Autodesk Inventor part; units mm, degrees
ref_plane "YZ Plane" through (0, 0, 0) normal (1, 0, 0) x (0, 1, 0)
ref_plane "XZ Plane" through (0, 0, 0) normal (0, 1, 0) x (-1, 0, 0)
ref_plane "XY Plane" through (0, 0, 0) normal (0, 0, 1) x (1, 0, 0)
sketch "Sketch1" plane through (0, 0, 0) normal (0, 0, 1) x (1, 0, 0)
  line L0 (0, 0) -> (25.4, 0)
  line L1 (25.4, 0) -> (25.4, 50.8)
  line L2 (25.4, 50.8) -> (0, 50.8)
  line L3 (0, 50.8) -> (0, 0)
  line L4 (1.5875, 49.2125) -> (23.8125, 49.2125)
  line L5 (23.8125, 49.2125) -> (23.8125, 1.5875)
  line L6 (23.8125, 1.5875) -> (1.5875, 1.5875)
  line L7 (1.5875, 1.5875) -> (1.5875, 49.2125)
  dimension "d0" = 25.4
  dimension "d1" = 50.8
  dimension "d2" = 1.5875
extrude "Extrusion1" add sketch "Sketch1" along normal blind 269.875
sketch "Sketch2" plane through (25.4, 0, 0) normal (1, 0, 0) x (0, 0, -1)
  line L0 (-269.875, 49.2125) -> (-269.875, 1.5875) construction
  line L1 (-269.875, 25.4) -> (-241.3, 25.4) construction
  circle A0 centre (-241.3, 25.4) radius 14.2875
  point P0 (0, 0)
  dimension "d20" = 28.575
  dimension "d21" = 28.575
sketch "Sketch4" plane through (0, 50.8, 0) normal (0, 1, 0) x (1, 0, 0)
  line L0 (1.5875, 0) -> (23.8125, 0) construction
  line L1 (12.7, 0) -> (12.7, -12.7) construction
  line L2 (12.7, -12.7) -> (12.7, -38.1) construction
  line L3 (12.7, -38.1) -> (12.7, -63.5) construction
  circle A0 centre (12.7, -12.7) radius 2.5797
  circle A1 centre (12.7, -38.1) radius 2.5797
  circle A2 centre (12.7, -63.5) radius 2.5797
  point P0 (0, 0)
  dimension "d14" = 12.7
  dimension "d15" = 25.4
  dimension "d16" = 25.4
  dimension "d17" = 5.1594
extrude "Extrusion4" cut sketch "Sketch4" against normal blind 68.2625
extrude "Extrusion5" cut sketch "Sketch2" against normal blind 25.4
sketch "Sketch5" plane through (25.4, 0, 0) normal (1, 0, 0) x (0, 0, -1)
  line L0 (0, 1.5875) -> (0, 49.2125) construction
  line L1 (0, 25.4) -> (-38.1, 25.4) construction
  line L2 (0, 25.4) -> (38.1, 25.4) construction
  line L3 (-38.1, 25.4) -> (-139.7, 25.4) construction
  circle A0 centre (-139.7, 25.4) radius 2.5797
  circle A1 centre (-38.1, 25.4) radius 2.5797
  circle A2 centre (-88.9, 25.4) radius 14.2875
  point P0 (0, 0)
  dimension "d24" = 38.1
  dimension "d25" = 180
  dimension "d26" = 101.6
  dimension "d27" = 5.1594
  dimension "d30" = 28.575
extrude "Extrusion7" cut sketch "Sketch5" against normal blind 25.4
sketch "Sketch7" plane through (0, 50.8, 0) normal (0, 1, 0) x (1, 0, 0)
  circle A0 centre (12.7, -63.5) radius 2.5797 construction
  line L0 (12.7, -63.5) -> (12.7, -88.9) construction
  circle A1 centre (12.7, -88.9) radius 2.5797
  point P0 (0, 0)
  dimension "d37" = 25.4
extrude "Extrusion9" cut sketch "Sketch7" against normal blind 66.675
sketch "Sketch8" plane through (0, 50.8, 0) normal (0, 1, 0) x (1, 0, 0)
  line L0 (23.8125, -269.875) -> (1.5875, -269.875) construction
  line L1 (12.7, -269.875) -> (12.7, -206.375) construction
  circle A0 centre (12.7, -206.375) radius 2.5797
  point P0 (0, 0)
  dimension "d40" = 63.5
  dimension "d41" = 5.1594
extrude "Extrusion10" cut sketch "Sketch8" against normal blind 66.675
The model under review builds one solid part; all positions refer to its coordinate system, in mm. A direction names the side the tool comes from. Round coordinates to 2 decimals unless told otherwise and drop trailing zeros. Write each loop counter-clockwise with the first axis right and the second up, starting at its lowest first coordinate (ties: lowest second). Pieces come first, ordered by that corner, then holes. Notation, with made-up numbers: (26.25, 45) - (66.25, 45) arc R19 cw to (66.25, 75) - close; hole circle Ø3 at (-38.5, 1). An arc over 180 degrees is marked (long way). One line per item, written item: value. Start each with the question number.
1. The part is to be moulded in two halves that separate along X. For faces 3 (the face through (14.087, 50.017, 35.925)), 4 (the face through (24.617, 23.83, 40.147)), 5 (the face through (12.364, 0.805, 203.817)), say which applies: released by +X, released by -X, zero draft, split by the parting line, or undercut.
2. Consider section D-D on z = 239. Write out the cut boundary in (x, y).
3. Consider section A-A on y = 6. Write out the cut boundary in (x, z) (1 decimal).
4. To check wall thickness, follow L1, parallel to Z at x = 12.7, y = 50.3 (3 decimals); L2, parallel to Y at x = 22.5, z = 156; L3, parallel to X at y = 0.85, z = 12.7. State the ranges of each line that lie inside material, in increasing order. Write a range as from..to.
5. Consider section B-B on x = 21. Write out the cut boundary in (y, z) (1 decimal).
6. Consider section C-C on z = 38.1. Write out the cut boundary in (x, y).
7. Machinability: for faces 1 (the face through (0.805, 23.83, 40.147)), 2 (the face through (1.588, 25, 133)), which of the approach directions +Z, -Z, +X, -X, +Y, -Y give a long, thin tool a straight path to every point of the face, cutting with its end or side? Answer none if there is none.
Checks:
1. face 3: undercut
1. face 4: zero draft
1. face 5: undercut
2. outline: (0, 0) - (25.4, 0) - (25.4, 11.3) - (23.81, 11.3) - (23.81, 1.59) - (1.59, 1.59) - (1.59, 11.3) - (0, 11.3) - close; (0, 39.5) - (1.59, 39.5) - (1.59, 49.21) - (23.81, 49.21) - (23.81, 39.5) - (25.4, 39.5) - (25.4, 50.8) - (0, 50.8) - close
3. outline: (0, 0) - (1.6, 0) - (1.6, 269.9) - (0, 269.9) - close; (23.8, 0) - (25.4, 0) - (25.4, 269.9) - (23.8, 269.9) - close
4. L1: z = 0..10.12, 15.28..35.52, 40.68..60.92, 66.08..86.32, 91.48..203.795, 208.955..269.875
4. L2: y = 0..1.59, 49.21..50.8
4. L3: x = 0..10.12, 15.28..25.4
5. outline: (0, 0) - (1.6, 0) - (1.6, 269.9) - (0, 269.9) - close; (49.2, 0) - (50.8, 0) - (50.8, 269.9) - (49.2, 269.9) - close
6. outline: (0, 0) - (10.12, 0) - (10.12, 1.59) - (1.59, 1.59) - (1.59, 22.82) - (0, 22.82) - close; (0, 27.98) - (1.59, 27.98) - (1.59, 49.21) - (10.12, 49.21) - (10.12, 50.8) - (0, 50.8) - close; (15.28, 0) - (25.4, 0) - (25.4, 22.82) - (23.81, 22.82) - (23.81, 1.59) - (15.28, 1.59) - close; (15.28, 49.21) - (23.81, 49.21) - (23.81, 27.98) - (25.4, 27.98) - (25.4, 50.8) - (15.28, 50.8) - close
7. face 1: +X, -X
7. face 2: +Z, -Z
